```python
from build123d import *

# Parameters (mm, degrees)
F0_W           = 30
F0_H           = 30
F1_DEPTH       = 15
F3_D           = 3.3
F3_CBORE_D     = 6
F3_CBORE_DEPTH = 3.3
F5_DEPTH       = 4


with BuildPart() as f1:
    # F0 (on Top) → F1 (new body)
    with BuildSketch(Plane.XY):
        Rectangle(F0_W, F0_H)
    extrude(amount=F1_DEPTH)

    # F3 (through all)
    with Locations(Plane.XY.offset(15)):
        with Locations((-8, 8), (8, -8)):
            CounterBoreHole(F3_D / 2, F3_CBORE_D / 2, F3_CBORE_DEPTH)

    # F4 (on face) → F5 (cut)
    with BuildSketch(Plane(origin=(0, 0, 0), x_dir=(1, 0, 0), z_dir=(0, 0, -1))):
        Polygon((-5, -9.732051), (-5, -6.267949), (-8, -4.535898), (-11, -6.267949), (-11, -9.732051), (-8, -11.464102), align=None)
        Polygon((8.025555, 4.535993), (11.012696, 6.290127), (10.987141, 9.754135), (7.974445, 11.464007), (4.987304, 9.709873), (5.012859, 6.245865), align=None)
    extrude(amount=-F5_DEPTH, mode=Mode.SUBTRACT)


solid = f1.part
```
CAD build for the part. Positions are in the model's coordinates, mm. A direction names the side the tool comes from. Round coordinates to 2 decimals unless told otherwise and drop trailing zeros. Order: outer loops, then holes, each group sorted by start corner. A loop starts at its lowest first (then second) coordinate and runs counter-clockwise, first axis right, second up. Notation, with made-up numbers: (31.25, -38.5) -> (88.25, -38.5) arc R31 cw to (88.25, -7.5) -> close; hole circle Ø9 at (-6.75, 21). An arc over 180 degrees is marked (long way). Write item = value, one per line.
(1) Cut at B-B (x = -7). Write the cut outline in (y, z).
Answers follow:
outline = (-15, 0) -> (5.11, 0) -> (5.11, 4) -> (6.69, 4) -> (6.69, 11.7) -> (5.17, 11.7) -> (5.17, 15) -> (-15, 15) -> close; (9.31, 4) -> (10.89, 4) -> (10.89, 0) -> (15, 0) -> (15, 15) -> (10.83, 15) -> (10.83, 11.7) -> (9.31, 11.7) -> close
(2) Pull direction Y, two halves, no side cores. Call faces 4 (the cylindrical face through (-6.784, 9.115, 7.796)), 5 (the flat face through (-11, 8, 2)), 6 (the flat face through (-15, 0, 7)), 7 (the flat face through (0, -15, 7)): +Y half, -Y half, draft (parallel to the pull), parting line (faces both ways), or undercut.
Answers follow:
face_4 = undercut
face_5 = undercut
face_6 = draft
face_7 = -Y half
(3) Drill centre lines: L1, parallel to Y at x = -8, z = 6.5; L2, parallel to Y at x = -8, z = 13.3; L3, parallel to X at y = -6.5, z = 11. Where is each one in solid material? Low to high.
Answers follow:
L1 = -15 to 6.35, 9.65 to 15
L2 = -15 to 5, 11 to 15
L3 = -15 to 7.31, 8.69 to 15
(4) Flat gauge pins, fed straight in: P1, Ø1.8, axis at x = 9, y = -8.5, coming from the -Z side; P2, Ø5.5, axis at x = 8, y = -8, coming from the +Z side. Where does each tip first touch, or does it go through?
Answers follow:
P1 = 4
P2 = 11.7
(5) 3-axis set-ups, long thin cutter, end or side, ignore diameter. For faces 1 (the flat face through (0, 15, 7)), 2 (the flat face through (6.5, -5.4, 2)), 3 (the cylindrical face through (10.86, -7.1, 13.37)): which of +Z, -Z, +X, -X, +Y, -Y reach the whole face in a straight line?
Answers follow:
face_1 = +Z, -Z, +X, -X, +Y
face_2 = -Z
face_3 = +Z
(6) Cut at A-A (y = 9). Write the cut outline in (x, z).
Answers follow:
outline = (-15, 0) -> (-11, 0) -> (-11, 4) -> (-9.31, 4) -> (-9.31, 11.7) -> (-10.83, 11.7) -> (-10.83, 15) -> (-15, 15) -> close; (-6.69, 4) -> (-5, 4) -> (-5, 0) -> (15, 0) -> (15, 15) -> (-5.17, 15) -> (-5.17, 11.7) -> (-6.69, 11.7) -> close
(7) Cut at C-C (y = -10.25). Write the cut outline in (x, z).
Answers follow:
outline = (-15, 0) -> (5.91, 0) -> (5.91, 4) -> (10.11, 4) -> (10.11, 0) -> (15, 0) -> (15, 15) -> (9.98, 15) -> (9.98, 11.7) -> (6.02, 11.7) -> (6.02, 15) -> (-15, 15) -> close
